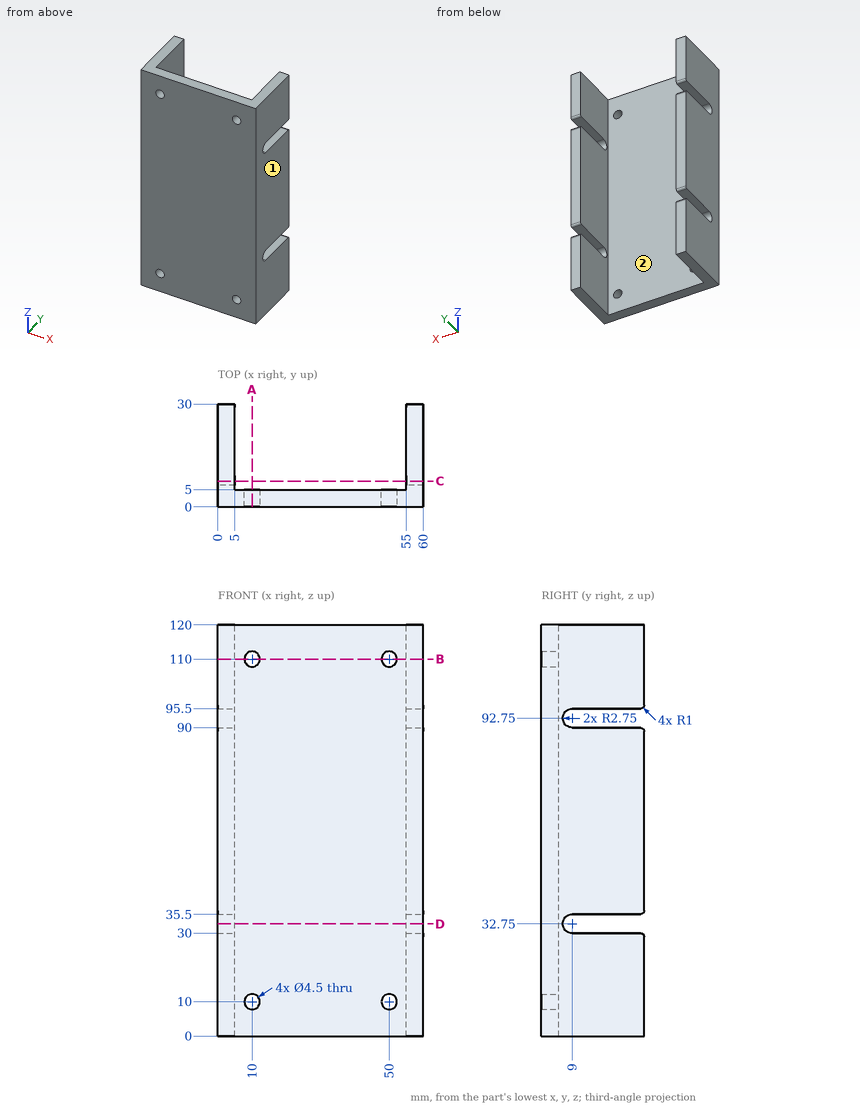
Drawing for the job (mm, zero at the part's lowest x, y, z). A direction names the side the tool comes from. Coordinates: 2 decimals unless noted, no trailing zeros. Write each loop counter-clockwise with the first axis right and the second up, starting at its lowest first coordinate (ties: lowest second). Pieces come first, ordered by that corner, then holes. Notation, with made-up numbers: (-24, -28.5) - (32, -28.5) arc R23 ccw to (32, 0.5) - close; hole circle Ø1 at (-32.75, 10). An arc over 180 degrees is marked (long way). Write each question's results on one line, items separated by ' | '. Start each with the question number.
1) Flat gauge pin, fed straight in: P1, Ø3, axis at x = 47.5, z = 106.5, coming from the +Y side. Where does the tip first touch, or does it go through?
2) 3-axis set-ups, long thin cutter, end or side, ignore diameter. For the marked faces 1 and 2: which of +Z, -Z, +X, -X, +Y, -Y reach the whole face in a straight line?
3) Cut at D-D (z = 32.75). Write the cut outline in (x, y), then the cut area to 4 significant figures.
4) Cut at B-B (z = 110). Write the cut outline in (x, y).
5) Cut at A-A (x = 10). Write the cut outline in (y, z), then the cut area to 3 significant figures.
6) Probe line 1 along Z through (x, y) = (50, 2.5); line 2 along X through (y, z) = (1.3, 110); line 3 along X through (y, z) = (26, 108.5). List the from-to ranges inside material, lowest first. Write a range as from..to.
7) Cut at C-C (y = 7.5). Write the cut outline in (x, z).
Returned:
1) P1: y = 5
2) face 1: +Z, -Z, +X, +Y, -Y | face 2: +Z, -Z, +Y
3) outline: (0, 0) - (60, 0) - (60, 6.25) - (55, 6.25) - (55, 5) - (5, 5) - (5, 6.25) - (0, 6.25) - close | area: 312.5 mm^2
4) outline: (0, 0) - (7.75, 0) - (7.75, 5) - (5, 5) - (5, 30) - (0, 30) - close; (12.25, 0) - (47.75, 0) - (47.75, 5) - (12.25, 5) - close; (52.25, 0) - (60, 0) - (60, 30) - (55, 30) - (55, 5) - (52.25, 5) - close
5) outline: (0, 0) - (5, 0) - (5, 7.75) - (0, 7.75) - close; (0, 12.25) - (5, 12.25) - (5, 107.75) - (0, 107.75) - close; (0, 112.25) - (5, 112.25) - (5, 120) - (0, 120) - close | area: 555 mm^2
6) line 1: 0..7.75, 12.25..107.75, 112.25..120 | line 2: 0..7.75, 12.25..47.75, 52.25..60 | line 3: 0..5, 55..60
7) outline: (0, 0) - (5, 0) - (5, 30.45) - (0, 30.45) - close; (0, 35.05) - (5, 35.05) - (5, 90.45) - (0, 90.45) - close; (0, 95.05) - (5, 95.05) - (5, 120) - (0, 120) - close; (55, 0) - (60, 0) - (60, 30.45) - (55, 30.45) - close; (55, 35.05) - (60, 35.05) - (60, 90.45) - (55, 90.45) - close; (55, 95.05) - (60, 95.05) - (60, 120) - (55, 120) - close
